Part model, mm, in its own coordinate system. Face numbers are marked on the shaded views. A direction names the side the tool comes from. Round coordinates to 2 decimals unless told otherwise and drop trailing zeros. Order: outer loops, then holes, each group sorted by start corner. A loop starts at its lowest first (then second) coordinate and runs counter-clockwise, first axis right, second up. Notation, with made-up numbers: (79.5, 49) -> (119.5, 49) arc R14 cw to (119.5, 74) -> close; hole circle Ø11 at (82, 79). An arc over 180 degrees is marked (long way). Use CSV: the item, a comma, the result in double quotes.
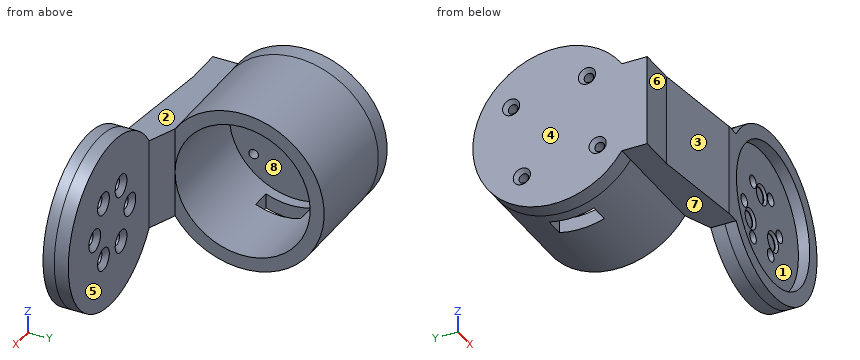
```python
from build123d import *

# Parameters (mm, degrees)
BOSS_EXTRUDE1_DEPTH                             = 5
CSK_FOR_M4_FLAT_HEAD_MACHINE_SCREW2_D           = 4.5
CSK_FOR_M4_FLAT_HEAD_MACHINE_SCREW2_CSINK_D     = 8
CSK_FOR_M4_FLAT_HEAD_MACHINE_SCREW2_CSINK_ANGLE = 90
SKETCH11_R                                      = 29
SKETCH11_R_2                                    = 24
BOSS_EXTRUDE2_DEPTH                             = 37
BOSS_EXTRUDE3_START                             = 6
BOSS_EXTRUDE3_DEPTH                             = 6
CSK_FOR_M3_FLAT_HEAD_MACHINE_SCREW1_D           = 3.4
CSK_FOR_M3_FLAT_HEAD_MACHINE_SCREW1_CSINK_D     = 6.1
CSK_FOR_M3_FLAT_HEAD_MACHINE_SCREW1_CSINK_ANGLE = 90
CUT_EXTRUDE1_REACH                              = 117.931
CUT_EXTRUDE1_END_RADIUS                         = 24
SKETCH15_W                                      = 7
SKETCH15_H                                      = 16
CUT_EXTRUDE2_START                              = -5
SKETCH17_R                                      = 2.9
CUT_EXTRUDE2_DEPTH                              = 1
CHAMFER1_SIZE                                   = 0.8
BOSS_EXTRUDE4_START                             = -43
BOSS_EXTRUDE4_DEPTH                             = 43
BOSS_EXTRUDE5_DEPTH                             = 16.28
BOSS_EXTRUDE6_START                             = 4
SKETCH21_R                                      = 30
SKETCH21_R_2                                    = 25
BOSS_EXTRUDE6_DEPTH                             = 4
BOSS_EXTRUDE7_DEPTH                             = 32.56


with BuildPart() as part:
    # Sketch1 → Boss-Extrude1 (new body)
    with BuildSketch(Plane(origin=(0, 0, 0), x_dir=(1, 0, 0), z_dir=(0, 1, 0))):
        with BuildLine():
            Line((-25.198444396, -16.28), (-72.198444396, -16.28))
            Line((-72.198444396, -16.28), (-72.198444396, 16.28))
            Line((-72.198444396, 16.28), (-25.198444396, 16.28))
            ThreePointArc((-25.198444396, 16.28), (30, 0), (-25.198444396, -16.28))
        make_face()
    extrude(amount=BOSS_EXTRUDE1_DEPTH)

    # CSK for M4 Flat Head Machine Screw2 (through all)
    with Locations(Plane(origin=(0, 5, 0), x_dir=(1, 0, 0), z_dir=(0, 1, 0))):
        with Locations((-6, 10.392304845), (-12, 0), (12, 0), (6, 10.392304845), (-6, -10.392304845), (6, -10.392304845)):
            CounterSinkHole(CSK_FOR_M4_FLAT_HEAD_MACHINE_SCREW2_D / 2, CSK_FOR_M4_FLAT_HEAD_MACHINE_SCREW2_CSINK_D / 2, counter_sink_angle=CSK_FOR_M4_FLAT_HEAD_MACHINE_SCREW2_CSINK_ANGLE)

    # Sketch11 → Boss-Extrude2 (add)
    with BuildSketch(Plane.ZY.offset(72.198444396)):
        with Locations((0, 33)):
            Circle(SKETCH11_R)
        with Locations((0, 33)):
            Circle(SKETCH11_R_2, mode=Mode.SUBTRACT)
    extrude(amount=-BOSS_EXTRUDE2_DEPTH)

    # Sketch12 → Boss-Extrude3 (add)
    with BuildSketch(Plane.ZY.offset(72.198444396).offset(BOSS_EXTRUDE3_START)):
        with BuildLine():
            Line((-16.28, 0), (16.28, 0))
            Line((16.28, 0), (16.28, 5))
            Line((16.28, 5), (7.549834435, 5))
            ThreePointArc((7.549834435, 5), (0, 62), (-7.549834435, 5))
            Line((-7.549834435, 5), (-16.28, 5))
            Line((-16.28, 5), (-16.28, 0))
        make_face()
    extrude(amount=-BOSS_EXTRUDE3_DEPTH)

    # CSK for M3 Flat Head Machine Screw1 (through all)
    with Locations(Plane.ZY.offset(78.198444396)):
        with Locations((-11.584939196, 17.626266432), (11.584939196, 48.373733568), (15.373733568, 21.415060804), (-15.373733568, 44.584939196)):
            CounterSinkHole(CSK_FOR_M3_FLAT_HEAD_MACHINE_SCREW1_D / 2, CSK_FOR_M3_FLAT_HEAD_MACHINE_SCREW1_CSINK_D / 2, counter_sink_angle=CSK_FOR_M3_FLAT_HEAD_MACHINE_SCREW1_CSINK_ANGLE)

    # Cut-Extrude1: up to this cylinder (the profile starts outside it)
    cut_extrude1_end = Plane(origin=(-64.698444, 33, 0), z_dir=(-1, 0, 0)) * Cylinder(CUT_EXTRUDE1_END_RADIUS, 284.862, mode=Mode.PRIVATE)
    # Sketch15 → Cut-Extrude1 (cut, up to the surface)
    with BuildSketch(Plane(origin=(0, 0, -29), x_dir=(-1, 0, 0), z_dir=(0, 0, -1)), mode=Mode.PRIVATE) as cut_extrude1_sk1:
        with Locations((64.698444396, 32.1)):
            Rectangle(SKETCH15_W, SKETCH15_H)
    cut_extrude1_tool1 = extrude(cut_extrude1_sk1.sketch, amount=-CUT_EXTRUDE1_REACH, mode=Mode.PRIVATE) - cut_extrude1_end
    add(cut_extrude1_tool1.solids().sort_by_distance((-64.698444, 32.1, -29))[0], mode=Mode.SUBTRACT)

    # Sketch17 → Cut-Extrude2 (cut)
    with BuildSketch(Plane(origin=(0, 5, 0), x_dir=(1, 0, 0), z_dir=(0, 1, 0)).offset(CUT_EXTRUDE2_START)):
        with Locations(Location((-7.664324823, 4.425, 0), (0, 0, 270))):
            Circle(SKETCH17_R)
        with Locations(Location((7.664324823, 4.425, 0), (0, 0, 270))):
            Circle(SKETCH17_R)
        with Locations(Location((0, -8.849999999, 0), (0, 0, 270))):
            Circle(SKETCH17_R)
    extrude(amount=CUT_EXTRUDE2_DEPTH, mode=Mode.SUBTRACT)

    # Chamfer1
    chamfer1_edges = [part.edges().sort_by_distance(p)[0] for p in [
        (7.664324823, 0, -7.325),
        (-7.664324823, 0, -7.325),
        (0, 0, 5.949999999),
    ]]
    chamfer(chamfer1_edges, length=CHAMFER1_SIZE)

    # Sketch19 → Boss-Extrude4 (add)
    with BuildSketch(Plane(origin=(-35.198444396, 0, 0), x_dir=(0, 0, -1), z_dir=(1, 0, 0)).offset(BOSS_EXTRUDE4_START)):
        with BuildLine():
            ThreePointArc((-7.549834435, 5), (-12.081674242, 6.636518676), (-16.28, 9.000800013))
            Line((-16.28, 9.000800013), (-16.28, 5))
            Line((-16.28, 5), (-7.549834435, 5))
        make_face()
        with BuildLine():
            Line((16.28, 5), (16.28, 9.000800013))
            ThreePointArc((16.28, 9.000800013), (12.081674242, 6.636518676), (7.549834435, 5))
            Line((7.549834435, 5), (16.28, 5))
        make_face()
    extrude(amount=BOSS_EXTRUDE4_DEPTH)

    # Sketch20 → Boss-Extrude5 (add, symmetric)
    with BuildSketch(Plane.XY):
        Polygon((-35.198444396, 9.000800013), (-25.198444396, 5), (-35.198444396, 5), align=None)
    extrude(amount=BOSS_EXTRUDE5_DEPTH, both=True)

    # Sketch21 → Boss-Extrude6 (add)
    with BuildSketch(Plane.XZ.offset(BOSS_EXTRUDE6_START)):
        with Locations(Location((0, 0, 0), (0, 0, 270))):
            Circle(SKETCH21_R)
        with Locations(Location((0, 0, 0), (0, 0, 270))):
            Circle(SKETCH21_R_2, mode=Mode.SUBTRACT)
    extrude(amount=-BOSS_EXTRUDE6_DEPTH)

    # Sketch22 → Boss-Extrude7 (add)
    with BuildSketch(Plane.XY.offset(16.28)):
        Polygon((-65, 0), (-25.198444396, 0), (-25, -4), (-30, -4), align=None)
    extrude(amount=-BOSS_EXTRUDE7_DEPTH)


solid = part.part
```
(1) Probe probe 1 along Z at (x, y) = (-6, 2); probe 2 along Z at (x, y) = (-61, 33); probe 3 along Y at (x, z) = (13, 12.5). List the from-to ranges inside material, lowest first. Write a range as [from, to].
Reply:
probe 1,"[-29.39, -12.64], [-8.14, 8.14], [12.64, 29.39]"
probe 2,"[-29, -24], [24, 29]"
probe 3,"[0, 5]"
(2) Cut at B-B, the plane x = 0. Give the cut face in (y, z), then the cut area to 3 significant figures.
Reply:
outline,"(-4, -30) -> (5, -30) -> (5, 30) -> (-4, 30) -> (-4, 25) -> (0, 25) -> (0, 12.55) -> (0.8, 11.75) -> (1, 11.75) -> (1, 5.95) -> (0.8, 5.95) -> (0, 5.15) -> (0, -25) -> (-4, -25) -> close"
area,"334 mm2"
(3) Pull direction Z, two halves, no side cores. Call the marked faces 1, 2 and 3: released by +Z, released by -Z, zero draft, split by the parting line, or undercut.
Reply:
face 1,"undercut"
face 2,"released by +Z"
face 3,"zero draft"
(4) Drop flat-ended pins along their axis: P1, Ø2, axis at x = -46, z = -9.5, coming from the +Y side; P2, Ø4, axis at x = -12, z = 0, coming from the +Y side; P3, Ø4, axis at y = 45.5, z = -18, coming from the +X side; P4, Ø2, axis at x = -3.5, z = -18, coming from the -Y side. Give the stop position or say it passes through.
Reply:
P1,"y = 60.73"
P2,"through"
P3,"x = -72.2"
P4,"y = 0"
(5) Which spindle directions (+Z, -Z, +X, -X, +Y, -Y) get a long thin tool onto all of the face, cutting with end or side? Do the marked faces 4, 5, 6, 7 and 8. Say none if no direction does.
Reply:
face 4,"+Z, -Z, -X, +Y, -Y"
face 5,"+Z, -Z, +X, +Y"
face 6,"+Z, -Z, -X, -Y"
face 7,"-Z, -X, -Y"
face 8,"+X"
(6) Cut at C-C, the plane x = -39. Give the cut face in (y, z), then the cut area to 3 significant figures.
Reply:
outline,"(-2.97, -16.28) -> (9, -16.28) arc R29 ccw (long way) to (9, 16.28) -> (-2.97, 16.28) -> close; hole circle Ø48 at (33, 0)"
area,"1,110 mm2"
(7) Cut at D-D, the plane y = 12.5. Give the cut face in (x, z), then the cut area to 3 significant figures.
Reply:
outline,"(-78.2, -20.51) -> (-35.2, -20.51) -> (-35.2, -12.48) -> (-72.2, -12.48) -> (-72.2, 12.48) -> (-35.2, 12.48) -> (-35.2, 20.51) -> (-78.2, 20.51) -> close"
area,"841 mm2"
(8) Cut at A-A, the plane y = 33. Give the cut face in (x, z).
Reply:
outline,"(-78.2, -29) -> (-68.2, -29) -> (-68.2, -24) -> (-72.2, -24) -> (-72.2, 24) -> (-35.2, 24) -> (-35.2, 29) -> (-78.2, 29) -> close; (-61.2, -29) -> (-35.2, -29) -> (-35.2, -24) -> (-61.2, -24) -> close"
